from build123d import *

# Parameters (mm, degrees)
SZKIC2_W                    = 74
SZKIC2_H                    = 226.2
DODANIE_WYCI_GNI_CIE1_DEPTH = 20
SZKIC3_W                    = 17.32
SZKIC3_H                    = 64
DODANIE_WYCI_GNI_CIE2_DEPTH = 69.53
SZKIC4_R                    = 3.999999999
WYTNIJ_WYCI_GNI_CIE1_DEPTH  = 20
SZKIC6_R                    = 4
WYTNIJ_WYCI_GNI_CIE3_DEPTH  = 21
SZKIC7_R                    = 4
WYTNIJ_WYCI_GNI_CIE4_DEPTH  = 20


with BuildPart() as part:
    # Szkic2 → Dodanie-wyciągnięcie1 (new body)
    with BuildSketch(Plane.XY.offset(-3.815865502)):
        with Locations((-0.134142184, -106.911615453)):
            Rectangle(SZKIC2_W, SZKIC2_H)
    extrude(amount=DODANIE_WYCI_GNI_CIE1_DEPTH)

    # Szkic3 → Dodanie-wyciągnięcie2 (add)
    with BuildSketch(Plane.ZY.offset(37.134142184)):
        with Locations((7.524134498, -188.011615453)):
            Rectangle(SZKIC3_W, SZKIC3_H)
    extrude(amount=DODANIE_WYCI_GNI_CIE2_DEPTH)

    # Szkic4 → Wytnij-wyciągnięcie1 (cut)
    with BuildSketch(Plane.XY.offset(16.184134498)):
        with Locations((-54.667677729, -191.906887131)):
            Circle(SZKIC4_R)
        with Locations((-98.667677729, -191.906887131)):
            Circle(SZKIC4_R)
    extrude(amount=-WYTNIJ_WYCI_GNI_CIE1_DEPTH, mode=Mode.SUBTRACT)

    # Szkic6 → Wytnij-wyciągnięcie3 (cut)
    with BuildSketch(Plane.XY.offset(-4.115865502)):
        with Locations((28.365857818, -199.506887131)):
            Circle(SZKIC6_R)
        with Locations((-28.634142182, -199.506887131)):
            Circle(SZKIC6_R)
        with Locations((-28.634142182, -154.506887131)):
            Circle(SZKIC6_R)
        with Locations((28.365857818, -154.506887131)):
            Circle(SZKIC6_R)
    extrude(amount=WYTNIJ_WYCI_GNI_CIE3_DEPTH, mode=Mode.SUBTRACT)

    # Szkic7 → Wytnij-wyciągnięcie4 (cut)
    with BuildSketch(Plane.XY.offset(-3.815865502)):
        with Locations((28.365857816, -14.506887131)):
            Circle(SZKIC7_R)
        with Locations((-28.634142184, -14.506887131)):
            Circle(SZKIC7_R)
        with Locations((-28.634142184, -59.506887131)):
            Circle(SZKIC7_R)
        with Locations((28.365857816, -59.506887131)):
            Circle(SZKIC7_R)
    extrude(amount=WYTNIJ_WYCI_GNI_CIE4_DEPTH, mode=Mode.SUBTRACT)


solid = part.part
Here's how the part is built. I have some questions about the finished solid (model axes, mm). A direction names the side the tool comes from. Coordinates: 2 decimals unless noted, no trailing zeros. Write each loop counter-clockwise with the first axis right and the second up, starting at its lowest first coordinate (ties: lowest second). Pieces come first, ordered by that corner, then holes.
1) If we section it at B-B (y = -166.5): List the corners of the cut face in (x, z) for me, plus the area to 3 significant figures.
Filled in:
outline: (-106.66, -1.14) - (-37.13, -1.14) - (-37.13, -3.82) - (36.87, -3.82) - (36.87, 16.18) - (-106.66, 16.18) - close
area: 2,680 mm2
2) Thinking about a two-plate mould opening in X: for faces 1 (the face through (25.42, -11.8, 6.04)), 2 (the face through (36.866, -108, 6)), 3 (the face through (-71, -156.012, 7)), which applies, +X half, -X half, draft (parallel to the pull), parting line (faces both ways), or undercut?
Filled in:
face 1: undercut
face 2: +X half
face 3: draft
3) If we section it at A-A (z = 10.75): Count the separate pieces of the cut face and the enclosed holes in it, plus the area to 3 significant figures.
Filled in:
separate pieces: 1
enclosed holes: 10
area: 20,700 mm2
4) Which directions (+Z, -Z, +X, -X, +Y, -Y) give clear straight access to the entire face, cutting with the end or side of a thin tool? Please do faces 4 (the face through (-29.501, -63.412, 6.044)), 5 (the face through (-71, -188, -1.136)).
Filled in:
face 4: +Z, -Z
face 5: -Z, -X, +Y, -Y
5) If I drill on line 1 (X direction, y = -194, z = 8); line 2 (X direction, y = -60.5, z = 10.25); line 3 (X direction, y = -106.5, z = 8.25), over which ranges is the centre line in solid material (lowest first)?
Filled in:
line 1: x = -106.66 to -102.08, -95.26 to -58.08, -51.26 to 36.87
line 2: x = -37.13 to -32.51, -24.76 to 24.49, 32.24 to 36.87
line 3: x = -37.13 to 36.87
6) If we section it at D-D (y = -116): List the corners of the cut face in (x, z) for me, plus the area to 3 significant figures.
Filled in:
outline: (-37.13, -3.82) - (36.87, -3.82) - (36.87, 16.18) - (-37.13, 16.18) - close
area: 1,480 mm2
7) If we section it at C-C (x = -88.5): List the corners of the cut face in (y, z) for me, plus the area to 3 significant figures.
Filled in:
outline: (-220.01, -1.14) - (-156.01, -1.14) - (-156.01, 16.18) - (-220.01, 16.18) - close
area: 1,110 mm2
8) I'm going to push flat-ended pins straight in: pin 1 (9 mm diameter, centred on x = -98.67, y = -191.91, fed in from -Z); pin 2 (10.5 mm diameter, centred on x = 28.37, y = -154.51, fed in from -Z); pin 3 (7 mm diameter, centred on x = 28.37, y = -59.51, fed in from +Z); pin 4 (5 mm diameter, centred on y = -135, z = 1.5, fed in from -X). Where does each tip first touch, or does it pass through?
Filled in:
pin 1: stops at z = -1.14
pin 2: stops at z = -3.82
pin 3: passes through
pin 4: stops at x = -37.13
